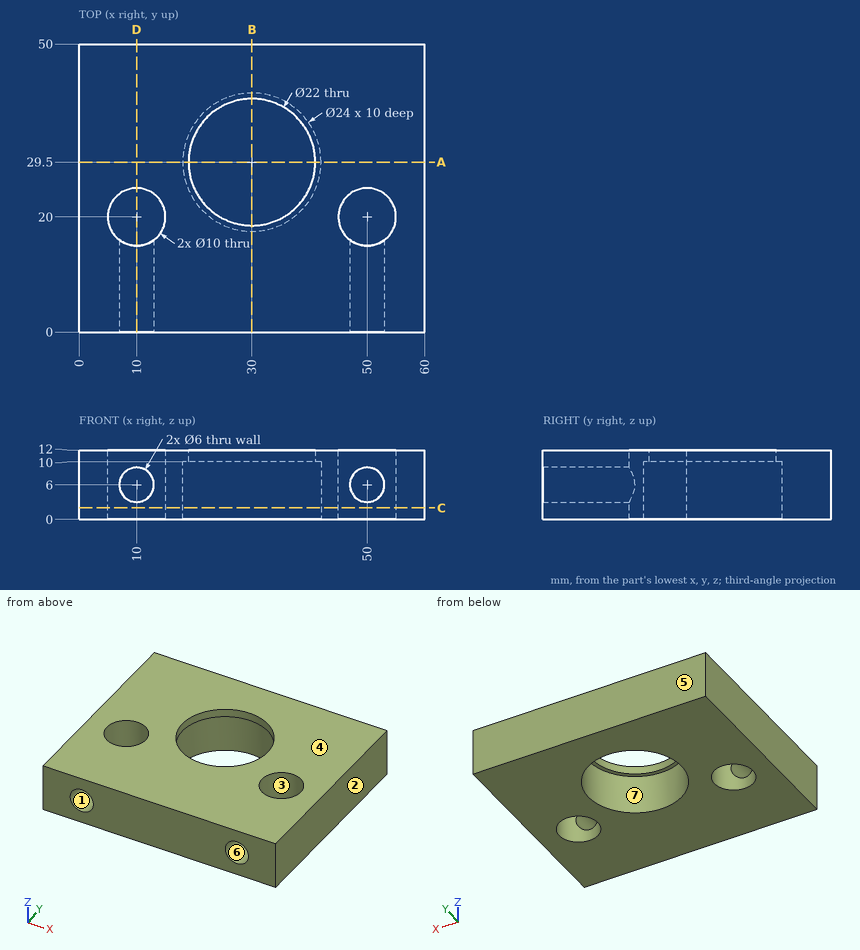
Job drawing, mm, ordinate dimensions from the low corner. One solid piece. A direction names the side the tool comes from. Give positions to 0.01 mm unless a question says otherwise; leave off trailing zeros. Write each loop counter-clockwise with the first axis right and the second up, starting at its lowest first coordinate (ties: lowest second). Pieces come first, ordered by that corner, then holes. Notation, with made-up numbers: (56.5, 83) - (103.5, 83) arc R23 cw to (103.5, 103) - close; hole circle Ø8 at (5, -30.5). An arc over 180 degrees is marked (long way). Answer as CSV lines item,"result".
1. Band-saw the part on A-A (y = 29.5). Write the cut outline in (x, z), and give its area (3 significant figures).
Responses:
outline,"(0, 0) - (18, 0) - (18, 10) - (19, 10) - (19, 12) - (0, 12) - close; (41, 10) - (42, 10) - (42, 0) - (60, 0) - (60, 12) - (41, 12) - close"
area,"436 mm2"
2. Pin check, flat tips, straight feed: pin 1 (12 mm diameter, centred on x = 26, y = 33.5, fed in from -Z); pin 2 (7 mm diameter, centred on x = 50, z = 6, fed in from -Y). Stop position of each tip, or through.
Responses:
pin 1,"stops at z = 10"
pin 2,"stops at y = 0"
3. Drill centre lines: L1, parallel to X at y = 12.25, z = 6; L2, parallel to Z at x = 50, y = 8; L3, parallel to X at y = 3, z = 7.75. Where is each one in solid material? Low to high. Write a range as [from, to].
Responses:
L1,"x = [0, 7], [13, 47], [53, 60]"
L2,"z = [0, 3], [9, 12]"
L3,"x = [0, 7.56], [12.44, 47.56], [52.44, 60]"
4. 3-axis set-ups, long thin cutter, end or side, ignore diameter. For the marked faces 5, 6 and 7: which of +Z, -Z, +X, -X, +Y, -Y reach the whole face in a straight line?
Responses:
face 5,"+Z, -Z, +X, -X, +Y"
face 6,"-Y"
face 7,"-Z"
5. Two-plate mould, pull along X, no slides. Class the marked faces 1, 2, 3 and 4: +X half, -X half, draft (parallel to the pull), parting line (faces both ways), or undercut.
Responses:
face 1,"undercut"
face 2,"+X half"
face 3,"undercut"
face 4,"draft"
6. Band-saw the part on B-B (x = 30). Write the cut outline in (y, z), and give its area (3 significant figures).
Responses:
outline,"(0, 0) - (17.5, 0) - (17.5, 10) - (18.5, 10) - (18.5, 12) - (0, 12) - close; (40.5, 10) - (41.5, 10) - (41.5, 0) - (50, 0) - (50, 12) - (40.5, 12) - close"
area,"316 mm2"
7. Band-saw the part on D-D (x = 10). Write the cut outline in (y, z).
Responses:
outline,"(0, 0) - (15, 0) - (15, 3) - (0, 3) - close; (0, 9) - (15, 9) - (15, 12) - (0, 12) - close; (25, 0) - (50, 0) - (50, 12) - (25, 12) - close"
8. Band-saw the part on C-C (z = 2). Write the cut outline in (x, y).
Responses:
outline,"(0, 0) - (60, 0) - (60, 50) - (0, 50) - close; hole circle Ø10 at (10, 20); hole circle Ø24 at (30, 29.5); hole circle Ø10 at (50, 20)"
